```python
from build123d import *

# Parameters (mm, degrees)
F0_R          = 82.164523
F0_R_2        = 6.35
F0_R_3        = 50.8
F1_DEPTH      = 15.875
F0_R_4        = 31.75
F2_DEPTH      = 44.45
F3_DEPTH      = 15.875
F3_DEPTH_BACK = 50.8


with BuildPart() as f1:
    # F0 (on Front) → F1 (new body)
    with BuildSketch(Plane.XZ):
        Circle(F0_R)
        with Locations((-60.491874, -34.925)):
            Circle(F0_R_2, mode=Mode.SUBTRACT)
        with Locations((0, -69.85)):
            Circle(F0_R_2, mode=Mode.SUBTRACT)
        with Locations((60.491874, -34.925)):
            Circle(F0_R_2, mode=Mode.SUBTRACT)
        with Locations((-60.491874, 34.925)):
            Circle(F0_R_2, mode=Mode.SUBTRACT)
        Circle(F0_R_3, mode=Mode.SUBTRACT)
        with Locations((60.491874, 34.925)):
            Circle(F0_R_2, mode=Mode.SUBTRACT)
        with Locations((0, 69.85)):
            Circle(F0_R_2, mode=Mode.SUBTRACT)
    extrude(amount=F1_DEPTH)

    # F0 (on Front) → F2 (join)
    with BuildSketch(Plane.XZ):
        Circle(F0_R_3)
        Circle(F0_R_4, mode=Mode.SUBTRACT)
    extrude(amount=F2_DEPTH)

    # F0 (on Front) → F3 (join, two sides)
    with BuildSketch(Plane.XZ) as f3_sk:
        with Locations((-60.491874, 34.925)):
            Circle(F0_R_2)
        with Locations((0, 69.85)):
            Circle(F0_R_2)
        with Locations((60.491874, 34.925)):
            Circle(F0_R_2)
        with Locations((60.491874, -34.925)):
            Circle(F0_R_2)
        with Locations((0, -69.85)):
            Circle(F0_R_2)
        with Locations((-60.491874, -34.925)):
            Circle(F0_R_2)
    extrude(amount=F3_DEPTH)
    extrude(f3_sk.sketch, amount=-F3_DEPTH_BACK)


solid = f1.part
```
Work out the finished part from the listing and answer in its coordinate system (mm). A direction names the side the tool comes from. Coordinates: 2 decimals unless noted, no trailing zeros. Order: outer loops, then holes, each group sorted by start corner. A loop starts at its lowest first (then second) coordinate and runs counter-clockwise, first axis right, second up. Notation, with made-up numbers: (17, 68) - (22, 68) arc R19 cw to (22, 88) - close; hole circle Ø9 at (-30.75, -21). An arc over 180 degrees is marked (long way). Answer as a JSON object with one key per item and string values.
1. Find section A-A on z = 0. Determine the outline of the cut face in (x, y) (3 decimals), plus the area to 3 significant figures.
Output values:
{"outline": "(-82.165, -15.875) - (-50.8, -15.875) - (-50.8, -44.45) - (-31.75, -44.45) - (-31.75, 0) - (-82.165, 0) - close; (31.75, -44.45) - (50.8, -44.45) - (50.8, -15.875) - (82.165, -15.875) - (82.165, 0) - (31.75, 0) - close", "area": "2,690 mm²"}
2. Find section B-B on x = 0. Determine the outline of the cut face in (y, z) (3 decimals), plus the area to 3 significant figures.
Output values:
{"outline": "(-44.45, -50.8) - (-15.875, -50.8) - (-15.875, -82.165) - (0, -82.165) - (0, -76.2) - (50.8, -76.2) - (50.8, -63.5) - (0, -63.5) - (0, -31.75) - (-44.45, -31.75) - close; (-44.45, 31.75) - (0, 31.75) - (0, 63.5) - (50.8, 63.5) - (50.8, 76.2) - (0, 76.2) - (0, 82.165) - (-15.875, 82.165) - (-15.875, 50.8) - (-44.45, 50.8) - close", "area": "3,980 mm²"}
3. Find section C-C on y = 24. Determine the outline of the cut face in (x, z) (3 decimals), plus the area to 3 significant figures.
Output values:
{"outline": "circle Ø12.7 at (-60.492, -34.925); circle Ø12.7 at (-60.492, 34.925); circle Ø12.7 at (0, -69.85); circle Ø12.7 at (0, 69.85); circle Ø12.7 at (60.492, -34.925); circle Ø12.7 at (60.492, 34.925)", "area": "760 mm²"}
4. Consider line 1 (Z direction, x = 0, y = -31.5); line 2 (Z direction, x = 0, y = -9); line 3 (X direction, y = -29.5, z = -1). Determine where each line is inside the solid, lowest interval first.
Output values:
{"line 1": "z = -50.8 to -31.75, 31.75 to 50.8", "line 2": "z = -82.16 to -31.75, 31.75 to 82.16", "line 3": "x = -50.79 to -31.73, 31.73 to 50.79"}
5. The mould has two halves that part along Z. Classify faces 1 (the face through (21.9, -44.45, 23.3)), 2 (the face through (-6.883, -21.914, -30.995)), 3 (the face through (78.37, -7.83, 24.68)): +Z half, -Z half, draft (parallel to the pull), parting line (faces both ways), or undercut.
Output values:
{"face 1": "draft", "face 2": "undercut", "face 3": "parting line"}
6. A tool of negligible diameter and unlimited length cuts with its end or side. For faces 4 (the face through (-61, 50.8, -35)), 5 (the face through (-66.836, 25.044, 35.204)), 6 (the face through (-38, -15.875, -35)), from which of +Z, -Z, +X, -X, +Y, -Y can it reach the whole face along a straight path? Write none if from no direction.
Output values:
{"face 4": "+Z, -Z, +X, -X, +Y", "face 5": "+Y", "face 6": "-Y"}
7. Each of these flat-tipped pins is pushed along its axis until it touches: P1, Ø10, axis at y = -19.5, z = -11.5, coming from the -X side; P2, Ø1, axis at y = -12.5, z = 39, coming from the -X side; P3, Ø3, axis at y = 16.5, z = -27, coming from the -X side; P4, Ø2, axis at y = -9.5, z = -39, coming from the +X side. Where does it stop, or does it pass through?
Output values:
{"P1": "stops at x = -81.77", "P2": "stops at x = -72.59", "P3": "passes through", "P4": "stops at x = 72.85"}
8. Find section D-D on z = -69.85. Determine the outline of the cut face in (x, y) (3 decimals), plus the area to 3 significant figures.
Output values:
{"outline": "(-43.266, -15.875) - (43.266, -15.875) - (43.266, 0) - (6.35, 0) - (6.35, 50.8) - (-6.35, 50.8) - (-6.35, 0) - (-43.266, 0) - close", "area": "2,020 mm²"}
